Can you work these out from the model? Positions are in its coordinate system, mm. Face numbers are marked on the shaded views. A direction names the side the tool comes from. Coordinates: 2 decimals unless noted, no trailing zeros. Loops run counter-clockwise (first coordinate to the right, second up) from the corner with the lowest first, then second, coordinate; pieces in that order, holes last. Notation, with made-up numbers: M -15.75,88 L 18.25,88 A30 ccw 18.25,123 Z; hole C 34.5,-27.75 d11. An arc over 180 degrees is marked long. Answer as a JSON object with one key per item and string values. Group by question number.
Item 1: Suppose I cut it at A-A (y = 0). Write out the boundary of the cut face in (x, z).
Item 2: We'd pull the mould along Y, two halves only. Please class the marked faces 5, 6 and 7: +Y half, -Y half, draft (parallel to the pull), parting line (faces both ways), or undercut.
Item 3: Suppose I cut it at C-C (z = 8.75). Count the separate pieces of the cut face and the enclosed holes in it, then the cut area to 3 significant figures.
Item 4: I'm going to push flat-ended pins straight in: pin 1 Ø6.5 at (x, z) = (6, 11) entering from +Y; pin 2 Ø3.5 at (x, y) = (-31, 3) entering from +Z; pin 3 Ø3.5 at (y, z) = (16.5, 6.5) entering from +X. Where does each tip first touch, or does it pass through?
Item 5: Suppose I cut it at B-B (x = 0). Write out the boundary of the cut face in (y, z), then the cut area to 3 significant figures.
Item 6: Which directions (+Z, -Z, +X, -X, +Y, -Y) give clear straight access to the entire face, cutting with the end or side of a thin tool? Please do the marked faces 1, 2, 3 and 4.
Item 7: If I drill on line 1 (X direction, y = 3, z = 13); line 2 (X direction, y = -4.5, z = 2.25); line 3 (Y direction, x = 23, z = 10.25), over which ranges is the centre line in solid material (lowest first)?
```python
from build123d import *

# Parameters (mm, degrees)
F0_R        = 41
F1_DEPTH    = 19
F3_DEPTH    = 17
F4_W        = 6
F4_H        = 11
F4_W_2      = 11
F4_H_2      = 16
F4_W_3      = 10.7800960541
F4_H_3      = 45.1917052269
F5_DEPTH    = 19.001
F7_START    = -12
F6_W        = 0.7
F6_H        = 5
F7_DEPTH    = 5
F8_W        = 16
F8_H        = 16
F9_DEPTH    = 1.82
F10_C1_SIZE = 2
F10_C2_SIZE = 1.9999
F11_W       = 12.5
F11_H       = 20
F12_DEPTH   = 5
F13_W       = 6
F13_H       = 35
F14_DEPTH   = 28.5


# Not quite as in the source:
# - a fillet or chamfer is up to 0.001 mm smaller than in the source, because OpenCascade refuses the exact size


with BuildPart() as f1:
    # F0 (on Top) → F1 (new body)
    with BuildSketch(Plane.XY):
        Circle(F0_R)
    extrude(amount=F1_DEPTH)

    # F2 (on face) → F3 (cut)
    with BuildSketch(Plane.XY.offset(19)):
        Polygon((39, 2.5), (39, 8), (1, 8), (1, -8), (39, -8), (39, -2.5), align=None)
        Polygon((-39, 8), (-39, 2.5), (-39, -2.5), (-39, -8), (-1, -8), (-1, 8), align=None)
        with BuildLine():
            Line((43, 2.5), (40.9237095093, 2.5))
            ThreePointArc((40.9237095093, 2.5), (40.9809229391, 1.2505818885), (41, 0))
            ThreePointArc((41, 0), (40.9809229391, -1.2505818885), (40.9237095093, -2.5))
            Line((40.9237095093, -2.5), (43, -2.5))
            Line((43, -2.5), (43, 2.5))
        make_face()
        with BuildLine():
            ThreePointArc((-40.9237095093, -2.5), (-41, 0), (-40.9237095093, 2.5))
            Line((-40.9237095093, 2.5), (-43, 2.5))
            Line((-43, 2.5), (-43, -2.5))
            Line((-43, -2.5), (-40.9237095093, -2.5))
        make_face()
        with BuildLine():
            Line((40.9237095093, 2.5), (39, 2.5))
            Line((39, 2.5), (39, -2.5))
            Line((39, -2.5), (40.9237095093, -2.5))
            ThreePointArc((40.9237095093, -2.5), (40.9809229391, -1.2505818885), (41, 0))
            ThreePointArc((41, 0), (40.9809229391, 1.2505818885), (40.9237095093, 2.5))
        make_face()
        with BuildLine():
            Line((-39, 2.5), (-40.9237095093, 2.5))
            ThreePointArc((-40.9237095093, 2.5), (-41, 0), (-40.9237095093, -2.5))
            Line((-40.9237095093, -2.5), (-39, -2.5))
            Line((-39, -2.5), (-39, 2.5))
        make_face()
    extrude(amount=-F3_DEPTH, mode=Mode.SUBTRACT)

    # F4 (on face) → F5 (cut, through all)
    with BuildSketch(Plane.XY.offset(19)):
        with Locations((-26.8149985671, 15.5)):
            Rectangle(F4_W, F4_H)
        with Locations((26.8149985671, 15.5)):
            Rectangle(F4_W, F4_H)
        with Locations((-5.5, 30.5270385295)):
            Rectangle(F4_W, F4_H)
        with Locations((5.5, 30.5270385295)):
            Rectangle(F4_W, F4_H)
        with Locations((-6.5, 0)):
            Rectangle(F4_W_2, F4_H_2)
        with Locations((6.5, 0)):
            Rectangle(F4_W_2, F4_H_2)
        with Locations((-45.090048027, 0)):
            Rectangle(F4_W_3, F4_H_3)
        with Locations((45.090048027, 0)):
            Rectangle(F4_W_3, F4_H_3)
    extrude(amount=-F5_DEPTH, mode=Mode.SUBTRACT)

    # F6 (on face) → F7 (join)
    with BuildSketch(Plane.XY.offset(19).offset(F7_START)):
        with Locations((-39.35, 0)):
            Rectangle(F6_W, F6_H)
        with Locations((39.35, 0)):
            Rectangle(F6_W, F6_H)
    extrude(amount=-F7_DEPTH)

    # F8 (on face) → F9 (join)
    with BuildSketch(Plane.XY.offset(2)):
        with Locations((-20, 0)):
            Rectangle(F8_W, F8_H)
        with Locations((20, 0)):
            Rectangle(F8_W, F8_H)
    extrude(amount=F9_DEPTH)

    # F10: chamfer of 2 on 2 edges, made by hand

    # F10_c1
    f10_c1_edges = [f1.edges().sort_by_distance(p)[0] for p in [
        (0, -41, 0),
    ]]
    chamfer(f10_c1_edges, length=F10_C1_SIZE)

    # F10_c2 (size 2 in the source; OpenCascade refuses exactly that, so slightly less here)
    f10_c2_edges = [f1.edges().sort_by_distance(p)[0] for p in [
        (0, 41, 0),
    ]]
    chamfer(f10_c2_edges, length=F10_C2_SIZE)

    # F11 (on face) → F12 (cut)
    with BuildSketch(Plane.XY.offset(19)):
        with Locations((0, -28.7845470011)):
            Rectangle(F11_W, F11_H)
    extrude(amount=-F12_DEPTH, mode=Mode.SUBTRACT)

    # F13 (on Right) → F14 (cut, symmetric)
    with BuildSketch(Plane.YZ):
        with Locations((-14.7845470011, -0.5)):
            Rectangle(F13_W, F13_H)
    extrude(amount=F14_DEPTH, both=True, mode=Mode.SUBTRACT)


solid = f1.part
```
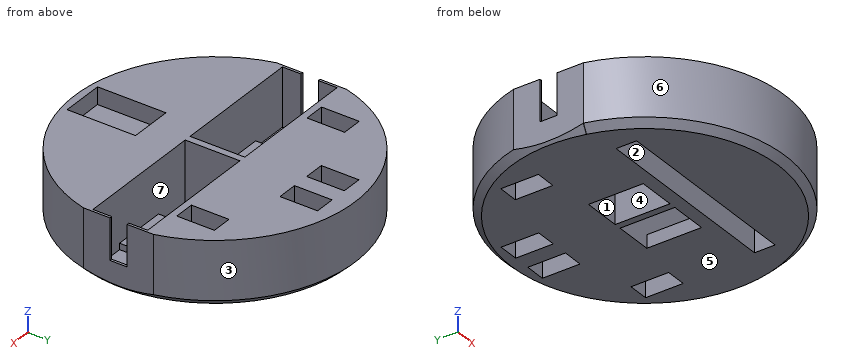
From the geometry:
{
 "1": {"outline": "M -39.7,0.7 L -39,0 L -12,0 L -12,3.82 L -28,3.82 L -28,2 L -39,2 L -39,7 L -39.7,7 Z; M -1,0 L 1,0 L 1,19 L -1,19 Z; M 12,0 L 39,0 L 39.7,0.7 L 39.7,7 L 39,7 L 39,2 L 28,2 L 28,3.82 L 12,3.82 Z"},
 "2": {"face 5": "draft", "face 6": "-Y half", "face 7": "undercut"},
 "3": {"separate pieces": "1", "enclosed holes": "5", "area": "3,420 mm2"},
 "4": {"pin 1": "y = 40.91", "pin 2": "z = 2", "pin 3": "x = 38.25"},
 "5": {"outline": "M -41,2 L -39,0 L -17.78,0 L -17.78,17 L -11.78,17 L -11.78,0 L 39,0 L 41,2 L 41,19 L -18.78,19 L -18.78,14 L -38.78,14 L -38.78,19 L -41,19 Z", "area": "1,350 mm2"},
 "6": {"face 1": "+Z", "face 2": "-Z", "face 3": "+Z, -Z, +Y", "face 4": "+Z, -Z"},
 "7": {"line 1": "-39.7 to -39, -1 to 1, 39 to 39.7", "line 2": "-39.7 to -39, -28 to -12, -1 to 1, 12 to 28, 39 to 39.7", "line 3": "-33.94 to -17.78, -11.78 to -8, 8 to 33.94"}
}
